Work out the finished part from the listing and answer in its coordinate system (mm). Give positions to 0.01 mm unless a question says otherwise; leave off trailing zeros. Write each loop counter-clockwise with the first axis right and the second up, starting at its lowest first coordinate (ties: lowest second). Pieces come first, ordered by that corner, then holes. Notation, with made-up numbers: (-8.75, 77.5) - (29.25, 77.5) arc R27 cw to (29.25, 103.5) - close; hole circle Ø3 at (84, 28.5). An arc over 180 degrees is marked (long way). Write each question's results on one line, items separated by ' | '. Start each with the question number.
from build123d import *

# Parameters (mm, degrees)
SKETCH2_R               = 1.375
SKETCH2_R_2             = 1
BOSS_EXTRUDE1_DEPTH     = 3
SCALE1_SCALE            = 2
SKETCH3_R               = 3
CUT_EXTRUDE1_DEPTH      = 168.69505013
CUT_EXTRUDE2_DEPTH      = 168.69505013
CUT_EXTRUDE2_DEPTH_BACK = 168.69505013


with BuildPart() as part:
    # Sketch2 → Boss-Extrude1 (new body)
    with BuildSketch(Plane.YZ):
        with BuildLine():
            ThreePointArc((52.261817642, 64.649681199), (55.722453046, 48.775220907), (69.655917155, 57.131838936))
            ThreePointArc((69.655917155, 57.131838936), (73.702355413, 73.305037878), (82.709556836, 87.334162909))
            ThreePointArc((82.709556836, 87.334162909), (79.248921432, 103.208623201), (65.315457322, 94.852005173))
            ThreePointArc((65.315457322, 94.852005173), (61.269019064, 78.67880623), (52.261817642, 64.649681199))
        make_face()
        with Locations(Location((75.281557454, 94.029297351, 0), (0, 0, 270))):
            Circle(SKETCH2_R, mode=Mode.SUBTRACT)
        with Locations(Location((59.689817023, 57.954546758, 0), (0, 0, 270))):
            Circle(SKETCH2_R_2, mode=Mode.SUBTRACT)
    extrude(amount=BOSS_EXTRUDE1_DEPTH)


with BuildPart() as part_1:
    # Scale1: scaled about (1.5, 67.462360836, 75.937951546)
    add(part.part.scale(SCALE1_SCALE).moved(Location((-1.5, -67.462360836, -75.937951546))))

    # Sketch3 → Cut-Extrude1 (cut, through all)
    with BuildSketch(Plane.YZ.offset(4.5)):
        with Locations(Location((83.100754073, 112.120643155, 0), (0, 0, 270))):
            Circle(SKETCH3_R)
    extrude(amount=-CUT_EXTRUDE1_DEPTH, mode=Mode.SUBTRACT)

    # Sketch4 → Cut-Extrude2 (cut, two sides: drawn at the far end of the back side and taken through both)
    with BuildSketch(Plane.YZ.offset(4.5).offset(-CUT_EXTRUDE2_DEPTH_BACK)):
        with BuildLine():
            ThreePointArc((63.168553809, 113.7660588), (55.075677293, 81.419660915), (37.061274447, 53.361410853))
            ThreePointArc((37.061274447, 53.361410853), (43.982545256, 21.612490269), (71.849473474, 38.325726326))
            ThreePointArc((71.849473474, 38.325726326), (79.94234999, 70.672124211), (97.956752836, 98.730374273))
            ThreePointArc((97.956752836, 98.730374273), (91.035482027, 130.479294857), (63.168553809, 113.7660588))
        make_face()
        with BuildLine():
            ThreePointArc((77.437713, 114.103057293), (85.469954791, 117.633073469), (88.436192443, 109.375994289))
            ThreePointArc((88.436192443, 109.375994289), (71.804815123, 74.18921939), (57.57219549, 37.96568591))
            ThreePointArc((57.57219549, 37.96568591), (49.557643799, 34.454607819), (46.56128374, 42.675467541))
            add(Edge.make_bspline(
                [(46.57708347, 42.706756435), (46.571822916, 42.696339697), (46.566556342, 42.685910072), (46.56128374, 42.675467541)],
                knots=[0.950044559, 0.950044559, 0.950044559, 0.950044559, 0.950284721, 0.950284721, 0.950284721, 0.950284721], degree=3))
            ThreePointArc((46.57708347, 42.706756435), (46.585069243, 42.722124357), (46.593054528, 42.737492531))
            ThreePointArc((46.593054528, 42.737492531), (63.286743628, 77.87078496), (77.437713, 114.103057293))
        make_face(mode=Mode.SUBTRACT)
    extrude(amount=CUT_EXTRUDE2_DEPTH + CUT_EXTRUDE2_DEPTH_BACK, mode=Mode.SUBTRACT)


solid = part_1.part
Q1. Given pin 1 (5.5 mm diameter, centred on y = 83.1, z = 112.12, fed in from -X); pin 2 (2 mm diameter, centred on x = 3, z = 86, fed in from -Y); pin 3 (1 mm diameter, centred on x = 1, z = 92.5, fed in from +Y); pin 4 (2 mm diameter, centred on x = -0.5, y = 75.5, fed in from -Z), each flat-ended and moving along its own axis, determine where each tip first touches the part or whether it passes through.
Q2. A cutting plane is placed at D-D, the plane y = 76. Write down the section's boundary in (x, z).
Q3. The mould has two halves that part along Z. Classify faces 1 (the cylindrical face through (1.46, 72.02, 74.69)), 2 (the cylindrical face through (1.54, 81.95, 109.35)), 3 (the cylindrical face through (1.458, 49.965, 40.405)), 4 (the cylindrical face through (1.458, 85.343, 117.686)): pulls with the +Z half, pulls with the -Z half, needs draft (parallel to the pull), parting line crosses it, or undercut.
Q4. A cutting plane is placed at C-C, the plane x = 3.5. Give the number of separate pieces and of enclosed holes in the cut face, and give its area (3 significant figures).
Q5. A cutting plane is placed at A-A, the plane y = 81. Write down the section's boundary in (x, z), and give its area (3 significant figures).
Q6. Consider L1, parallel to Y at x = 2.25, z = 39; L2, parallel to Z at x = 0.5, y = 53.5; L3, parallel to Y at x = 1.5, z = 55. Determine where each line is inside the solid, lowest interval first.
Q7. A cutting plane is placed at B-B, the plane z = 58. Write down the section's boundary in (x, y), and give its area (3 significant figures).
Result:
1) pin 1: passes through | pin 2: stops at y = 66.31 | pin 3: stops at y = 80.34 | pin 4: stops at z = 80.33
2) outline: (-1.5, 83.66) - (4.5, 83.66) - (4.5, 110.05) - (-1.5, 110.05) - close
3) face 1: pulls with the -Z half | face 2: undercut | face 3: undercut | face 4: parting line crosses it
4) separate pieces: 1 | enclosed holes: 2 | area: 874 mm2
5) outline: (-1.5, 94.39) - (4.5, 94.39) - (4.5, 109.98) - (-1.5, 109.98) - close; (-1.5, 114.26) - (4.5, 114.26) - (4.5, 117.74) - (-1.5, 117.74) - close | area: 114 mm2
6) L1: y = 46 to 50.17, 53.67 to 57.94 | L2: z = 34.18 to 38.75, 41.19 to 56.5 | L3: y = 52.77 to 63.92
7) outline: (-1.5, 54.22) - (4.5, 54.22) - (4.5, 65.1) - (-1.5, 65.1) - close | area: 65.2 mm2
